Design review of the part shown in the three views and the two pictorial views. Dimensions are in mm from the part's minimum x, y and z. A direction names the side the tool comes from. Coordinates: 2 decimals unless noted, no trailing zeros. Loops run counter-clockwise (first coordinate to the right, second up) from the corner with the lowest first, then second, coordinate; pieces in that order, holes last. Notation, with made-up numbers: (45, 28.5) -> (51, 28.5) arc R26 cw to (51, 53.5) -> close; hole circle Ø1 at (-19, 10). An arc over 180 degrees is marked (long way). One line per item, written item: value.
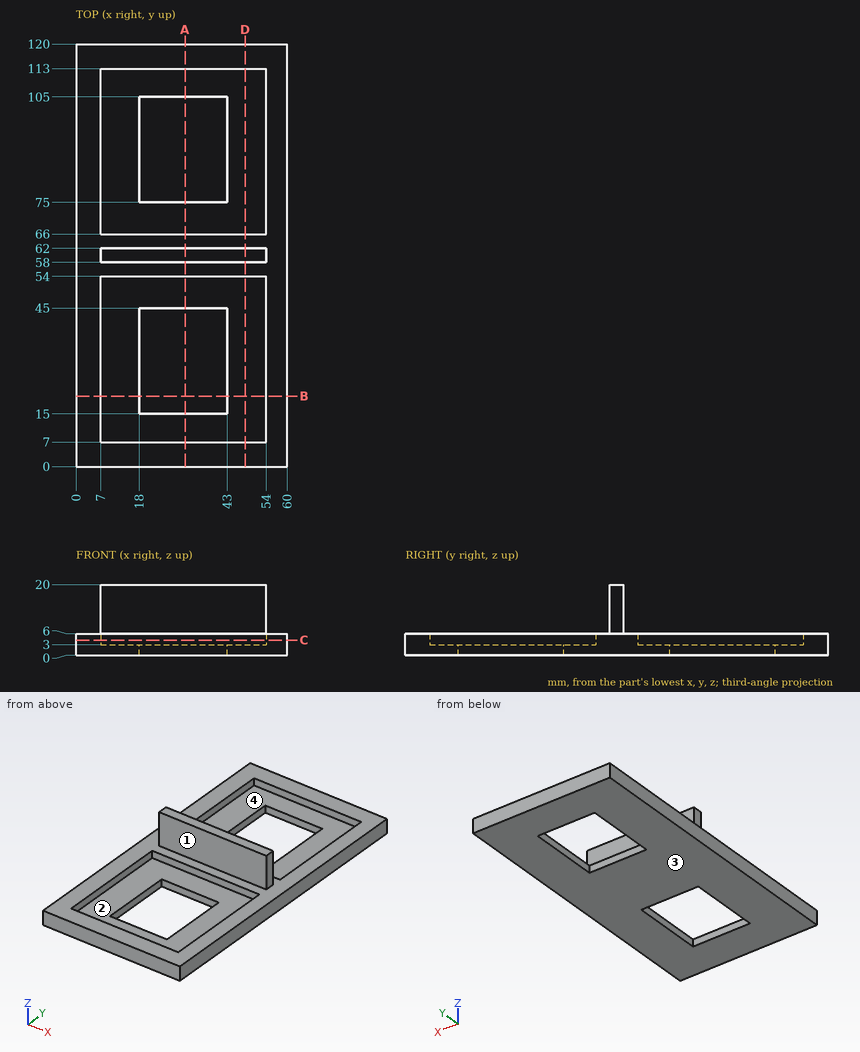
1. Take a section at A-A, the plane x = 31. Give the boundary of the cut face in (y, z), and give its area (3 significant figures).
Return value:
outline: (0, 0) -> (15, 0) -> (15, 3) -> (7, 3) -> (7, 6) -> (0, 6) -> close; (45, 0) -> (75, 0) -> (75, 3) -> (66, 3) -> (66, 6) -> (62, 6) -> (62, 20) -> (58, 20) -> (58, 6) -> (54, 6) -> (54, 3) -> (45, 3) -> close; (105, 0) -> (120, 0) -> (120, 6) -> (113, 6) -> (113, 3) -> (105, 3) -> close
area: 314 mm2
2. Take a section at C-C, the plane z = 4.25. Give the boundary of the cut face in (x, y), and give its area (3 significant figures).
Return value:
outline: (0, 0) -> (60, 0) -> (60, 120) -> (0, 120) -> close; hole (7, 7) -> (54, 7) -> (54, 54) -> (7, 54) -> close; hole (7, 66) -> (54, 66) -> (54, 113) -> (7, 113) -> close
area: 2,780 mm2
3. Take a section at B-B, the plane y = 20. Give the boundary of the cut face in (x, z), and give its area (3 significant figures).
Return value:
outline: (0, 0) -> (18, 0) -> (18, 3) -> (7, 3) -> (7, 6) -> (0, 6) -> close; (43, 0) -> (60, 0) -> (60, 6) -> (54, 6) -> (54, 3) -> (43, 3) -> close
area: 144 mm2
4. To check wall thickness, follow probe 1 along Y at (x, z) = (45.5, 4.75); probe 2 along X at (y, z) = (42.5, 1.25); probe 3 along Y at (x, z) = (35.5, 7.5). State the ranges of each line that lie inside material, in increasing order. Write a range as from..to.
Return value:
probe 1: y = 0..7, 54..66, 113..120
probe 2: x = 0..18, 43..60
probe 3: y = 58..62
5. The part is to be moulded in two halves that separate along X. For the marked faces 1 and 2, say which applies: pulls with the +X half, pulls with the -X half, needs draft (parallel to the pull), parting line crosses it, or undercut.
Return value:
face 1: needs draft
face 2: undercut
6. Insertion check: pin 1 Ø8 at (x, y) = (37.5, 79.5) entering from +Z; pin 2 Ø4 at (x, z) = (15, 16.5) entering from -Y; pin 3 Ø6 at (x, y) = (26, 16) entering from +Z; pin 4 Ø4 at (x, z) = (8.5, 17.5) entering from +Y. Each pin has a flat end and moves straight along its axis. Give the tip position at first contact, or say it passes through.
Return value:
pin 1: passes through
pin 2: stops at y = 58
pin 3: stops at z = 3
pin 4: stops at y = 62
7. Take a section at D-D, the plane x = 48. Give the boundary of the cut face in (y, z).
Return value:
outline: (0, 0) -> (120, 0) -> (120, 6) -> (113, 6) -> (113, 3) -> (66, 3) -> (66, 6) -> (62, 6) -> (62, 20) -> (58, 20) -> (58, 6) -> (54, 6) -> (54, 3) -> (7, 3) -> (7, 6) -> (0, 6) -> close
8. For the marked faces 3 and 4, list the 3-axis set-ups (+Z, -Z, +X, -X, +Y, -Y) from which the entire face can be reached by the end or side of a thin tool; tool diameter is ignored.
Return value:
face 3: -Z, +X, -X, +Y, -Y
face 4: +Z
